from build123d import *

# Parameters (mm, degrees)
BOSS_EXTRU_3_DEPTH      = 80
ESQUISSE17_R            = 3.5
ENL_V_MAT_EXTRU_4_DEPTH = 7
ESQUISSE18_R            = 3.5
ENL_V_MAT_EXTRU_5_DEPTH = 7.298921418
CHANFREIN5_SIZE         = 2
CONG_1_R                = 4
CONG_2_R                = 1


with BuildPart() as part:
    # Esquisse16 → Boss.-Extru.3 (new body)
    with BuildSketch(Plane.XY):
        Polygon((0, 0), (10, 0), (10, -8), (50, -8), (50, 0), (60, 0), (60, -12), (80, -12), (80, -18), (-20, -18.298921418), (-20, -12.298921418), (0, -12.298921418), align=None)
    extrude(amount=-BOSS_EXTRU_3_DEPTH)

    # Esquisse17 → Enlèv. mat.-Extru.4 (cut, through all)
    with BuildSketch(Plane(origin=(0, -12.298921418, 0), x_dir=(1, 0, 0), z_dir=(0, 1, 0))):
        with Locations((-10, 65)):
            Circle(ESQUISSE17_R)
        with Locations((-10, 40)):
            Circle(ESQUISSE17_R)
        with Locations((-10, 15)):
            Circle(ESQUISSE17_R)
    extrude(amount=-ENL_V_MAT_EXTRU_4_DEPTH, mode=Mode.SUBTRACT)

    # Esquisse18 → Enlèv. mat.-Extru.5 (cut, through all)
    with BuildSketch(Plane(origin=(0, -12, 0), x_dir=(1, 0, 0), z_dir=(0, 1, 0))):
        with Locations((70, 65)):
            Circle(ESQUISSE18_R)
        with Locations((70, 40)):
            Circle(ESQUISSE18_R)
        with Locations((70, 15)):
            Circle(ESQUISSE18_R)
    extrude(amount=-ENL_V_MAT_EXTRU_5_DEPTH, mode=Mode.SUBTRACT)

    # Chanfrein5
    chanfrein5_edges = [part.edges().sort_by_distance(p)[0] for p in [
        (60, -12, -40),
        (0, -12.298921418, -40),
    ]]
    chamfer(chanfrein5_edges, length=CHANFREIN5_SIZE)

    # Congé1
    cong_1_edges = [part.edges().sort_by_distance(p)[0] for p in [
        (10, -8, -40),
        (50, -8, -40),
    ]]
    fillet(cong_1_edges, radius=CONG_1_R)

    # Congé2
    cong_2_edges = [part.edges().sort_by_distance(p)[0] for p in [
        (5, 0, 0),
        (55, 0, 0),
        (0, 0, -40),
        (10, 0, -40),
        (50, 0, -40),
        (60, 0, -40),
        (55, 0, -80),
        (5, 0, -80),
    ]]
    fillet(cong_2_edges, radius=CONG_2_R)


solid = part.part
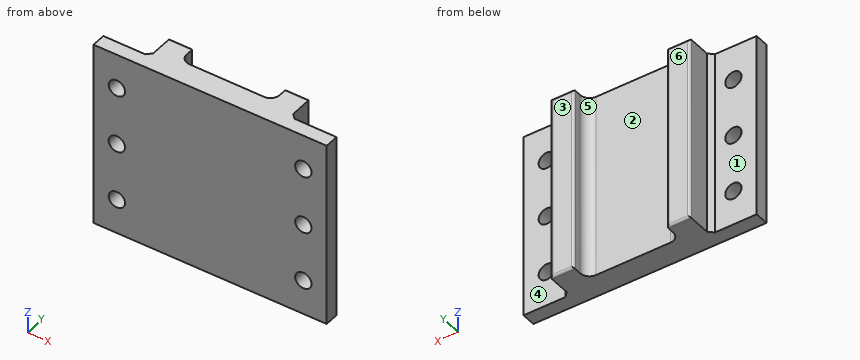
Can you work these out from the model? Positions are in its coordinate system, mm. Face numbers are marked on the shaded views. A direction names the side the tool comes from. Round coordinates to 2 decimals unless told otherwise and drop trailing zeros. Order: outer loops, then holes, each group sorted by start corner. A loop starts at its lowest first (then second) coordinate and runs counter-clockwise, first axis right, second up. Notation, with made-up numbers: M 83,-26.75 L 92,-26.75 A31 ccw 92,12.25 Z; hole C -35.75,-7.5 d1. An arc over 180 degrees is marked long. Use a Markdown table: item, result.
1) Imagine slicing it at D-D (z = -40). List the corners of the cut face in (x, y) for me, then the cut area to 3 significant figures.
Geometry says:
| item | result |
|---|---|
| outline | M -20,-18.3 L -13.5,-18.28 L -13.5,-12.3 L -20,-12.3 Z; M -6.5,-18.26 L 66.5,-18.04 L 66.5,-12 L 62,-12 L 60,-10 L 60,-1 A1 ccw 59,0 L 51,0 A1 ccw 50,-1 L 50,-4 A4 cw 46,-8 L 14,-8 A4 cw 10,-4 L 10,-1 A1 ccw 9,0 L 1,0 A1 ccw 0,-1 L 0,-10.3 L -2,-12.3 L -6.5,-12.3 Z; M 73.5,-18.02 L 80,-18 L 80,-12 L 73.5,-12 Z |
| area | 935 mm² |
2) I'm going to push flat-ended pins straight in: P1, Ø3.5, axis at y = -2.5, z = -41.5, coming from the +X side; P2, Ø3, axis at y = -6, z = -24.5, coming from the -X side; P3, Ø5.5, axis at x = 68.5, z = -24, coming from the +Y side. Where does each tip first touch, or does it pass through?
Geometry says:
| item | result |
|---|---|
| P1 | stops at x = 60 |
| P2 | stops at x = 0 |
| P3 | stops at y = -12 |
3) If we mould it in two halves opening along X, with no side actions, what happens to the marked faces 5 and 6? For each: +X half, -X half, draft (parallel to the pull), parting line (faces both ways), or undercut.
Geometry says:
| item | result |
|---|---|
| face 5 | undercut |
| face 6 | draft |
4) If I drill on line 1 along X through (y, z) = (-16.75, -65); line 2 along Z through (x, y) = (70, -16.5); line 3 along X through (y, z) = (-4, -13), over which ranges is the centre line in solid material (lowest first)?
Geometry says:
| item | result |
|---|---|
| line 1 | x = -20 to -13.5, -6.5 to 66.5, 73.5 to 80 |
| line 2 | z = -80 to -68.5, -61.5 to -43.5, -36.5 to -18.5, -11.5 to 0 |
| line 3 | x = 0 to 10, 50 to 60 |
5) Imagine slicing it at B-B (y = -14). List the corners of the cut face in (x, z) for me.
Geometry says:
| item | result |
|---|---|
| outline | M -20,-80 L 80,-80 L 80,0 L -20,0 Z; hole C -10,-65 d7; hole C -10,-40 d7; hole C -10,-15 d7; hole C 70,-65 d7; hole C 70,-40 d7; hole C 70,-15 d7 |
6) Imagine slicing it at C-C (z = -27). List the corners of the cut face in (x, y) for me, then the cut area to 3 significant figures.
Geometry says:
| item | result |
|---|---|
| outline | M -20,-18.3 L 80,-18 L 80,-12 L 62,-12 L 60,-10 L 60,-1 A1 ccw 59,0 L 51,0 A1 ccw 50,-1 L 50,-4 A4 cw 46,-8 L 14,-8 A4 cw 10,-4 L 10,-1 A1 ccw 9,0 L 1,0 A1 ccw 0,-1 L 0,-10.3 L -2,-12.3 L -20,-12.3 Z |
| area | 1,020 mm² |
7) Imagine slicing it at A-A (x = -10). List the corners of the cut face in (y, z) for me.
Geometry says:
| item | result |
|---|---|
| outline | M -18.27,-80 L -12.3,-80 L -12.3,-68.5 L -18.27,-68.5 Z; M -18.27,-61.5 L -12.3,-61.5 L -12.3,-43.5 L -18.27,-43.5 Z; M -18.27,-36.5 L -12.3,-36.5 L -12.3,-18.5 L -18.27,-18.5 Z; M -18.27,-11.5 L -12.3,-11.5 L -12.3,0 L -18.27,0 Z |
8) On a 3-axis mill with a long thin cutter (end or side, diameter ignored), from which of +Z, -Z, +X, -X, +Y, -Y can I reach the whole of each face in a straight line? I mean the marked faces 1, 2, 3 and 4. Say none if no direction works.
Geometry says:
| item | result |
|---|---|
| face 1 | +Z, -Z, -X, +Y |
| face 2 | +Z, -Z, +Y |
| face 3 | +Z, -Z, +X, -X, +Y |
| face 4 | +Z, -Z, +X, +Y |
